from build123d import *

# Parameters (mm, degrees)
BLANKSKE_W         = 150
BLANKSKE_H         = 12
BLANK_DEPTH        = 10
TOOTHCUTSIM_DEPTH  = 151.811140172
TEETHCUTS_COUNT    = 25
TEETHCUTS_PITCH    = 6.2831853
SKETCH1_W          = 35
SKETCH1_H          = 10
CUT_EXTRUDE1_DEPTH = 3.5
CUT_EXTRUDE2_REACH = 152.811
SKETCH2_R          = 2.5


with BuildPart() as part:
    # BlankSke → Blank (new body)
    with BuildSketch(Plane.XY):
        with Locations((75, 6)):
            Rectangle(BLANKSKE_W, BLANKSKE_H)
    extrude(amount=-BLANK_DEPTH)

    # TooCutSkeSim → ToothCutSim (cut, through all)
    with BuildSketch(Plane.XY):
        Polygon((0.861870739, 7.5), (-0.861870739, 7.5), (-2.508981637, 12.0254), (2.508981637, 12.0254), align=None)
    toothcutsim = extrude(amount=-TOOTHCUTSIM_DEPTH, mode=Mode.SUBTRACT)

    # TeethCuts: ToothCutSim ×25
    with Locations(*[(i * TEETHCUTS_PITCH, 0, 0) for i in range(1, TEETHCUTS_COUNT)]):
        add(toothcutsim, mode=Mode.SUBTRACT)

    # Sketch1 → Cut-Extrude1 (cut)
    with BuildSketch(Plane.XZ):
        with Locations((75, -5)):
            Rectangle(SKETCH1_W, SKETCH1_H)
    extrude(amount=-CUT_EXTRUDE1_DEPTH, mode=Mode.SUBTRACT)

    # Cut-Extrude2: up to this face of the body (flat: up to its plane)
    cut_extrude2_end = Plane(part.part.faces().sort_by_distance((141.37166925, 12, -5))[0])
    # Sketch2 → Cut-Extrude2 (cut, up to the picked face)
    with BuildSketch(Plane.XZ, mode=Mode.PRIVATE) as cut_extrude2_sk1:
        with Locations(Location((6, -5, 0), (0, 0, 270))):
            Circle(SKETCH2_R)
    cut_extrude2_tool1 = split(extrude(cut_extrude2_sk1.sketch, amount=-CUT_EXTRUDE2_REACH, mode=Mode.PRIVATE), bisect_by=cut_extrude2_end, keep=Keep.BOTH, mode=Mode.PRIVATE)
    # Sketch2 → Cut-Extrude2 (cut, up to the picked face)
    with BuildSketch(Plane.XZ, mode=Mode.PRIVATE) as cut_extrude2_sk2:
        with Locations(Location((144, -5, 0), (0, 0, 261.984352652))):
            Circle(SKETCH2_R)
    cut_extrude2_tool2 = split(extrude(cut_extrude2_sk2.sketch, amount=-CUT_EXTRUDE2_REACH, mode=Mode.PRIVATE), bisect_by=cut_extrude2_end, keep=Keep.BOTH, mode=Mode.PRIVATE)
    add(cut_extrude2_tool1.solids().sort_by(Axis((6, 0, -5), (0, 1, 0)))[0], mode=Mode.SUBTRACT)
    add(cut_extrude2_tool2.solids().sort_by(Axis((144, 0, -5), (0, 1, 0)))[0], mode=Mode.SUBTRACT)


solid = part.part
Part model, mm, in its own coordinate system. Coordinates: 2 decimals unless noted, no trailing zeros. Write each question's results on one line, items separated by ' | '. Start each with the question number.
Q1. Slice it at A-A on y = 9.5. Give the number of separate pieces and of enclosed holes in the cut face, and give its area (3 significant figures).
Q2. Probe line 1 along X through (y, z) = (5, -5); line 2 along X through (y, z) = (3, -5.75); line 3 along Z through (x, y) = (6, 3.75). List the from-to ranges inside material, lowest first.
Q3. Two-plate mould, pull along X, no slides. Class faces 1 (the flat face through (0, 4, -5)), 2 (the flat face through (74, 5, -10)), 3 (the flat face through (57.5, 2, -5)): +X half, -X half, draft (parallel to the pull), parting line (faces both ways), or undercut.
Q4. Drop flat-ended pins along their axis: pin 1 Ø0.9 at (x, z) = (6.5, -1) entering from +Y; pin 2 Ø6 at (x, z) = (6, -5) entering from +Y; pin 3 Ø3 at (x, z) = (80.5, -9) entering from -Y. Give the stop position or say it passes through.
Answer:
1) separate pieces: 24 | enclosed holes: 0 | area: 735 mm2
2) line 1: x = 0 to 3.5, 8.5 to 141.5, 146.5 to 150 | line 2: x = 0 to 3.62, 8.38 to 57.5, 92.5 to 141.62, 146.38 to 150 | line 3: z = -10 to -7.5, -2.5 to 0
3) face 1: -X half | face 2: draft | face 3: undercut
4) pin 1: stops at y = 7.5 | pin 2: stops at y = 12 | pin 3: stops at y = 3.5
